Autodesk Inventor part; units mm, degrees
ref_plane "YZ Plane" through (0, 0, 0) normal (1, 0, 0) x (0, 1, 0)
ref_plane "XZ Plane" through (0, 0, 0) normal (0, 1, 0) x (-1, 0, 0)
ref_plane "XY Plane" through (0, 0, 0) normal (0, 0, 1) x (1, 0, 0)
sketch "Szkic1" plane through (0, 0, 0) normal (0, 0, 1) x (1, 0, 0)
  line L0 (6, 4) -> (-6, 4)
  line L1 (-6, 4) -> (-6, 2.5)
  line L2 (-6, 2.5) -> (-4.5, 2.5)
  line L3 (-4.5, 2.5) -> (-4.5, 1)
  line L4 (-4.5, 1) -> (-6, 1)
  line L5 (-6, 4) -> (-6, 2.5)
  line L6 (-6, 1) -> (-6, -1)
  line L7 (6, 4) -> (6, 2.5)
  line L8 (6, 2.5) -> (4.5, 2.5)
  line L9 (4.5, 2.5) -> (4.5, 1)
  line L10 (4.5, 1) -> (6, 1)
  line L11 (6, -1) -> (6, 1)
  line L12 (6, 2.5) -> (6, 4)
  line L13 (0, 9) -> (-13.5, 9)
  line L14 (0, 9) -> (13.5, 9)
  line L15 (-13.5, 9) -> (-13.5, -1)
  line L16 (13.5, -1) -> (13.5, 9)
  line L17 (-13.5, -1) -> (-6, -1)
  line L18 (6, -1) -> (13.5, -1)
  point P0 (0, 0)
  point P1 (0, 0)
extrude "Wyciągnięcie proste1" add sketch "Szkic1" along normal blind 32.4
sketch "Szkic2" plane through (-13.5, 9, 0) normal (0, 1, 0) x (1, 0, 0)
  line L0 (27, 0) -> (0, 0)
  line L1 (0, 0) -> (0, -32.4)
  line L2 (27, -32.4) -> (0, -32.4)
  line L3 (27, 0) -> (27, -32.4)
  line L4 (0, 0) -> (0, -32.4)
  line L5 (27, -32.4) -> (0, 0)
  line L6 (0, -32.4) -> (27, 0)
  line L7 (13.5, -6.2) -> (5, -6.2)
  line L8 (3.5, -7.7) -> (3.5, -24.7)
  line L9 (5, -26.2) -> (22, -26.2)
  line L10 (23.5, -24.7) -> (23.5, -7.7)
  line L11 (22, -6.2) -> (13.5, -6.2)
  circle A0 centre (3.5, -26.2) radius 1.5
  circle A1 centre (3.5, -6.2) radius 1.5
  circle A2 centre (23.5, -26.2) radius 1.5
  circle A3 centre (23.5, -6.2) radius 1.5
  point P0 (13.5, 0)
  dimension "d12" = 3
  dimension "d13" = 3
  dimension "d14" = 3
  dimension "d15" = 3
extrude "Wyciągnięcie proste2" cut sketch "Szkic2" against normal blind 3.5 contours A3 L6 | L6 A3 | A1 L5 | L5 A1 | A2 L5 | L5 A2 | A0 L6 | L6 A0
thread "Gwint1"
thread "Gwint2"
thread "Gwint3"
thread "Gwint4"
sketch "Szkic3" plane through (0, 0, 32.4) normal (0, 0, 1) x (1, 0, 0)
  line L0 (6, 4) -> (6, 2.5)
  line L1 (6, 2.5) -> (4.5, 2.5)
  line L2 (4.5, 2.5) -> (4.5, 1)
  line L3 (4.5, 1) -> (6, 1)
  line L4 (6, 1) -> (6, -1)
  line L5 (6, -1) -> (13.5, -1)
  line L6 (13.5, -1) -> (13.5, 9)
  line L7 (13.5, 9) -> (-13.5, 9)
  line L8 (-13.5, 9) -> (-13.5, -1)
  line L9 (-13.5, -1) -> (-6, -1)
  line L10 (-6, -1) -> (-6, 1)
  line L11 (-6, 1) -> (-4.5, 1)
  line L12 (-4.5, 1) -> (-4.5, 2.5)
  line L13 (-4.5, 2.5) -> (-6, 2.5)
  line L14 (-6, 2.5) -> (-6, 4)
  line L15 (-6, 4) -> (6, 4)
  line L16 (-13.5, -1) -> (-13, -1)
  line L17 (-13.5, -1) -> (-6, -1)
  line L18 (-13, -1) -> (-13, 8.5)
  line L19 (13.5, -1) -> (13, -1)
  line L20 (6, -1) -> (13.5, -1)
  line L21 (13, -1) -> (13, 8.5)
  line L22 (13, 8.5) -> (-13, 8.5)
  point P0 (0, 0)
  dimension "d26" = 0.5
  dimension "d27" = 0.5
extrude "Wyciągnięcie proste3" add sketch "Szkic3" along normal blind 5 contours L15 L14 L13 L12 L11 L10 L9 L18 L22 L21 L5 L4 L3 L2 L1 L0
sketch "Szkic4" plane through (0, 0, 37.4) normal (0, 0, 1) x (1, 0, 0)
  line L0 (6, 4) -> (6, 2.5)
  line L1 (6, 2.5) -> (4.5, 2.5)
  line L2 (4.5, 2.5) -> (4.5, 1)
  line L3 (4.5, 1) -> (6, 1)
  line L4 (6, 1) -> (6, -1)
  line L5 (6, -1) -> (13, -1)
  line L6 (13, -1) -> (13, 8.5)
  line L7 (13, 8.5) -> (-13, 8.5)
  line L8 (-13, 8.5) -> (-13, -1)
  line L9 (-13, -1) -> (-6, -1)
  line L10 (-6, -1) -> (-6, 1)
  line L11 (-6, 1) -> (-4.5, 1)
  line L12 (-4.5, 1) -> (-4.5, 2.5)
  line L13 (-4.5, 2.5) -> (-6, 2.5)
  line L14 (-6, 2.5) -> (-6, 4)
  line L15 (-6, 4) -> (6, 4)
  line L16 (-13, -1) -> (-12.5, -1)
  line L17 (-13.5, -1) -> (-6, -1)
  line L18 (-12.5, -1) -> (-12.5, 8)
  line L19 (13, -1) -> (12.5, -1)
  line L20 (6, -1) -> (13.5, -1)
  line L21 (12.5, -1) -> (12.5, 8)
  line L22 (12.5, 8) -> (-12.5, 8)
  point P0 (0, 0)
extrude "Wyciągnięcie proste4" add sketch "Szkic4" along normal blind 1.5 contours L15 L14 L13 L12 L11 L10 L9 L18 L22 L21 L5 L4 L3 L2 L1 L0
sketch "Szkic5" plane through (0, 0, 0) normal (0, 0, -1) x (-1, 0, 0)
  line L0 (-6, -1) -> (-13, -1)
  line L1 (-6, 4) -> (-6, 2.5)
  line L2 (6, 4) -> (-6, 4)
  line L3 (6, 2.5) -> (6, 4)
  line L4 (4.5, 2.5) -> (6, 2.5)
  line L5 (4.5, 1) -> (4.5, 2.5)
  line L6 (6, 1) -> (4.5, 1)
  line L7 (6, -1) -> (6, 1)
  line L8 (-6, -1) -> (-13, -1)
  line L9 (-6, 1) -> (-6, -1)
  line L10 (-4.5, 1) -> (-6, 1)
  line L11 (-4.5, 2.5) -> (-4.5, 1)
  line L12 (-6, 2.5) -> (-4.5, 2.5)
  line L13 (13.5, -1) -> (6, -1)
  line L14 (6, -1) -> (13, -1)
  line L15 (-6, 4) -> (-6, 2.5)
  line L16 (6, 4) -> (-6, 4)
  line L17 (6, 2.5) -> (6, 4)
  line L18 (4.5, 2.5) -> (6, 2.5)
  line L19 (4.5, 1) -> (4.5, 2.5)
  line L20 (6, 1) -> (4.5, 1)
  line L21 (6, -1) -> (6, 1)
  line L22 (13.5, -1) -> (6, -1)
  line L23 (13.5, 9) -> (13.5, -1)
  line L24 (-13.5, 9) -> (13.5, 9)
  line L25 (-13.5, -1) -> (-13.5, 9)
  line L26 (-6, -1) -> (-13.5, -1)
  line L27 (-6, 1) -> (-6, -1)
  line L28 (-4.5, 1) -> (-6, 1)
  line L29 (-4.5, 2.5) -> (-4.5, 1)
  line L30 (-6, 2.5) -> (-4.5, 2.5)
  line L31 (-13.5, -1) -> (-13.5, 9)
  line L32 (-13.5, 9) -> (-13, 9)
  line L33 (-13, -1) -> (-13, 8.5)
  line L34 (-13, 9) -> (-13, -1)
  line L35 (13.5, 9) -> (13, 9)
  line L36 (-13.5, 9) -> (13.5, 9)
  line L37 (13, 9) -> (13, -1)
  line L38 (-13, 9) -> (-13, 8.5)
  line L39 (13, 8.5) -> (-13, 8.5)
  line L40 (-13, 8.5) -> (13, 8.5)
  point P0 (0, 0)
  dimension "d45" = 0.5
  dimension "d46" = 0.5
  dimension "d47" = 0.5
  dimension "d49" = 26
extrude "Wyciągnięcie proste5" add sketch "Szkic5" along normal blind 5 contours L0 L33 L39 L37 L13 L7 L6 L5 L4 L3 L2 L1 L12 L11 L10 L9
sketch "Szkic7" plane through (0, 0, -5) normal (0, 0, -1) x (-1, 0, 0)
  line L0 (-13, -1) -> (-6, -1)
  line L1 (-6, -1) -> (-6, 1)
  line L2 (-6, 1) -> (-4.5, 1)
  line L3 (-4.5, 1) -> (-4.5, 2.5)
  line L4 (-4.5, 2.5) -> (-6, 2.5)
  line L5 (-6, 2.5) -> (-6, 4)
  line L6 (-6, 4) -> (6, 4)
  line L7 (6, 4) -> (6, 2.5)
  line L8 (6, 2.5) -> (4.5, 2.5)
  line L9 (4.5, 2.5) -> (4.5, 1)
  line L10 (4.5, 1) -> (6, 1)
  line L11 (6, 1) -> (6, -1)
  line L12 (6, -1) -> (13, -1)
  line L13 (-6, -1) -> (-12.5, -1)
  line L14 (-13, -1) -> (-12.5, -1)
  line L15 (-12.5, -1) -> (-12.5, 8)
  line L16 (13, -1) -> (12.5, -1)
  line L17 (6, -1) -> (13, -1)
  line L18 (12.5, -1) -> (12.5, 8)
  line L19 (12.5, 8) -> (12.5, -1)
  line L20 (-12.5, -1) -> (-12.5, 8)
  line L21 (12.5, 8) -> (-12.5, 8)
  point P0 (0, 0)
  dimension "d53" = 25
  dimension "d54" = 9
  dimension "d55" = 9
extrude "Wyciągnięcie proste6" add sketch "Szkic7" along normal blind 1.5
sketch "Szkic8" plane through (-13.5, 9, 0) normal (0, 1, 0) x (1, 0, 0)
  circle A0 centre (23.5, -6.2) radius 1.5
  circle A1 centre (23.5, -26.2) radius 1.5
  circle A2 centre (3.5, -6.2) radius 1.5
  circle A3 centre (3.5, -26.2) radius 1.5
  line L0 (27, 0) -> (0, 0)
  line L1 (0, 0) -> (0, -32.4)
  line L2 (27, -32.4) -> (0, -32.4)
  line L3 (27, 0) -> (27, -32.4)
  line L4 (27, 0) -> (27, -32.4)
  line L5 (27, 0) -> (20, 0)
  line L6 (20, 0) -> (20, -32.4)
  line L7 (0, -32.4) -> (7, -32.4)
  line L8 (27, -32.4) -> (0, -32.4)
  line L9 (7, -32.4) -> (7, 0)
  point P0 (13.5, 0)
  dimension "d58" = 7
  dimension "d59" = 7
extrude "Wyciągnięcie proste7" cut sketch "Szkic8" against normal blind 0.25 contours L6 L2 L9 L0
properties part number "Wózek MGN12H"
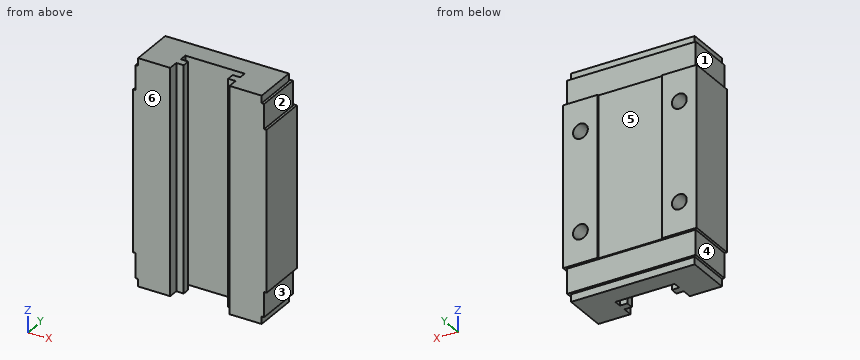
Part model, mm, in its own coordinate system. Face numbers are marked on the shaded views. A direction names the side the tool comes from. Round coordinates to 2 decimals unless told otherwise and drop trailing zeros. Write each loop counter-clockwise with the first axis right and the second up, starting at its lowest first coordinate (ties: lowest second). Pieces come first, ordered by that corner, then holes. Notation, with made-up numbers: (-17.75, 41.25) - (-3.75, 41.25) arc R28 cw to (-3.75, 60.25) - close; hole circle Ø6 at (18, -38). An arc over 180 degrees is marked (long way). Use CSV: the item, a comma, the result in double quotes.
Item 1: Slice it at C-C, the plane z = 30. Write the cut outline in (x, y), then the cut area to 3 significant figures.
Results list:
outline,"(-13.5, -1) - (-6, -1) - (-6, 1) - (-4.5, 1) - (-4.5, 2.5) - (-6, 2.5) - (-6, 4) - (6, 4) - (6, 2.5) - (4.5, 2.5) - (4.5, 1) - (6, 1) - (6, -1) - (13.5, -1) - (13.5, 9) - (6.5, 9) - (6.5, 8.75) - (-6.5, 8.75) - (-6.5, 9) - (-13.5, 9) - close"
area,"211 mm²"
Item 2: Slice it at A-A, the plane x = 5.5. Write the cut outline in (y, z), then the cut area to 3 significant figures.
Results list:
outline,"(1, -6.5) - (2.5, -6.5) - (2.5, 38.9) - (1, 38.9) - close; (4, -6.5) - (8, -6.5) - (8, -5) - (8.5, -5) - (8.5, 0) - (8.75, 0) - (8.75, 32.4) - (8.5, 32.4) - (8.5, 37.4) - (8, 37.4) - (8, 38.9) - (4, 38.9) - close"
area,"279 mm²"
Item 3: Pull direction X, two halves, no side cores. Call the marked faces 4, 5 and 6: pulls with the +X half, pulls with the -X half, needs draft (parallel to the pull), parting line crosses it, or undercut.
Results list:
face 4,"pulls with the -X half"
face 5,"undercut"
face 6,"needs draft"
Item 4: Slice it at D-D, the plane x = 10. Write the cut outline in (y, z).
Results list:
outline,"(-1, -6.5) - (8, -6.5) - (8, -5) - (8.5, -5) - (8.5, 0) - (9, 0) - (9, 4.7) - (5.5, 4.7) - (5.5, 7.7) - (9, 7.7) - (9, 24.7) - (5.5, 24.7) - (5.5, 27.7) - (9, 27.7) - (9, 32.4) - (8.5, 32.4) - (8.5, 37.4) - (8, 37.4) - (8, 38.9) - (-1, 38.9) - close"
Item 5: Wall check: L1, parallel to Z at x = -10, y = 6.4; L2, parallel to X at y = 8.15, z = 26.2; L3, parallel to Z at x = 10, y = 8.1. Give the ranges that are in metal, low to high.
Results list:
L1,"z = -6.5 to 4.7, 7.7 to 24.7, 27.7 to 38.9"
L2,"x = -13.5 to -11.5, -8.5 to 8.5, 11.5 to 13.5"
L3,"z = -5 to 4.7, 7.7 to 24.7, 27.7 to 37.4"
Item 6: Tool access for the marked faces 1, 2 and 3: list every direction of +Z, -Z, +X, -X, +Y, -Y with a clear straight run to the whole face (end or side of a thin tool).
Results list:
face 1,"+Z, -X, +Y, -Y"
face 2,"+Z, +X, +Y, -Y"
face 3,"-Z, +X, +Y, -Y"
Item 7: Flat gauge pins, fed straight in: P1, Ø6, axis at x = 10.5, z = 6, coming from the +Y side; P2, Ø2.5, axis at x = -2, z = 34, coming from the +Y side; P3, Ø1.2, axis at y = 2, z = 38.5, coming from the -X side; P4, Ø1.6, axis at x = -0.5, z = -6, coming from the +Y side. Where does each tip first touch, or does it go through?
Results list:
P1,"stops at y = 9"
P2,"stops at y = 8.5"
P3,"stops at x = -12.5"
P4,"stops at y = 8"
Item 8: Slice it at B-B, the plane y = -0.5. Write the cut outline in (x, z).
Results list:
outline,"(-13.5, 0) - (-13, 0) - (-13, -5) - (-12.5, -5) - (-12.5, -6.5) - (-6, -6.5) - (-6, 38.9) - (-12.5, 38.9) - (-12.5, 37.4) - (-13, 37.4) - (-13, 32.4) - (-13.5, 32.4) - close; (6, -6.5) - (12.5, -6.5) - (12.5, -5) - (13, -5) - (13, 0) - (13.5, 0) - (13.5, 32.4) - (13, 32.4) - (13, 37.4) - (12.5, 37.4) - (12.5, 38.9) - (6, 38.9) - close"
